CAD build for the part. Positions are in the model's coordinates, mm. A direction names the side the tool comes from. Coordinates: 2 decimals unless noted, no trailing zeros. Order: outer loops, then holes, each group sorted by start corner. A loop starts at its lowest first (then second) coordinate and runs counter-clockwise, first axis right, second up. Notation, with made-up numbers: M 18.5,51.25 L 69.5,51.25 A23 cw 69.5,79.25 Z; hole C 71,-25.5 d9. An arc over 180 degrees is marked long. One line per item, written item: value.
from build123d import *

# Parameters (mm, degrees)
SKETCH1_W                = 66.5
SKETCH1_H                = 180
BOSS_EXTRUDE1_DEPTH      = 180
SKETCH3_W                = 160
SKETCH3_H                = 160
CUT_EXTRUDE1_DEPTH       = 180
SKETCH8_W                = 66.5
SKETCH8_H                = 40
BOSS_EXTRUDE2_DEPTH      = 5
SKETCH10_W               = 66.5
SKETCH10_H               = 40
BOSS_EXTRUDE3_DEPTH      = 5
SKETCH5_R                = 14
CUT_EXTRUDE3_DEPTH       = 10
CUT_EXTRUDE5_DEPTH       = 5
CUT_EXTRUDE6_START       = -5
CUT_EXTRUDE6_DEPTH       = 5
SKETCH12_W               = 66.5
SKETCH12_H               = 40
BOSS_EXTRUDE8_DEPTH      = 5
SKETCH15_R               = 14
CUT_EXTRUDE7_DEPTH       = 200
SKETCH7_R                = 14
CORTE_EXTRUS_O1_DEPTH    = 10
SKETCH13_W               = 66.5
SKETCH13_H               = 40
RESSALTO_EXTRUS_O1_DEPTH = 5


with BuildPart() as part:
    # Sketch1 → Boss-Extrude1 (new body)
    with BuildSketch(Plane.XY):
        with Locations((33.25, 90)):
            Rectangle(SKETCH1_W, SKETCH1_H)
    extrude(amount=BOSS_EXTRUDE1_DEPTH)

    # Sketch3 → Cut-Extrude1 (cut)
    with BuildSketch(Plane.ZY):
        with Locations((90, 90)):
            Rectangle(SKETCH3_W, SKETCH3_H)
    extrude(amount=-CUT_EXTRUDE1_DEPTH, mode=Mode.SUBTRACT)

    # Sketch8 → Boss-Extrude2 (add)
    with BuildSketch(Plane.XY.offset(10)):
        with Locations((33.25, 150)):
            Rectangle(SKETCH8_W, SKETCH8_H)
    extrude(amount=BOSS_EXTRUDE2_DEPTH)

    # Sketch10 → Boss-Extrude3 (add)
    with BuildSketch(Plane(origin=(0, 0, 170), x_dir=(-1, 0, 0), z_dir=(0, 0, -1))):
        with Locations((-33.25, 150)):
            Rectangle(SKETCH10_W, SKETCH10_H)
    extrude(amount=BOSS_EXTRUDE3_DEPTH)

    # Sketch5 → Cut-Extrude3 (cut)
    with BuildSketch(Plane(origin=(0, 180, 0), x_dir=(1, 0, 0), z_dir=(0, 1, 0))):
        with Locations(Location((49.5, -90, 0), (0, 0, 270))):
            Circle(SKETCH5_R)
    extrude(amount=-CUT_EXTRUDE3_DEPTH, mode=Mode.SUBTRACT)

    # Sketch9 → Cut-Extrude5 (cut)
    with BuildSketch(Plane.XY.offset(15)):
        with BuildLine():
            Line((60.5, 164.5), (7.5, 164.5))
            ThreePointArc((7.5, 164.5), (5.378679656, 163.621320344), (4.5, 161.5))
            Line((4.5, 161.5), (4.5, 138.5))
            ThreePointArc((4.5, 138.5), (5.378679656, 136.378679656), (7.5, 135.5))
            Line((7.5, 135.5), (60.5, 135.5))
            ThreePointArc((60.5, 135.5), (62.621320344, 136.378679656), (63.5, 138.5))
            Line((63.5, 138.5), (63.5, 161.5))
            ThreePointArc((63.5, 161.5), (62.621320344, 163.621320344), (60.5, 164.5))
        make_face()
    extrude(amount=-CUT_EXTRUDE5_DEPTH, mode=Mode.SUBTRACT)

    # Sketch11 → Cut-Extrude6 (cut)
    with BuildSketch(Plane(origin=(0, 0, 165), x_dir=(-1, 0, 0), z_dir=(0, 0, -1)).offset(CUT_EXTRUDE6_START)):
        with BuildLine():
            Line((-60.5, 164.5), (-7, 164.5))
            ThreePointArc((-7, 164.5), (-4.878679656, 163.621320344), (-4, 161.5))
            Line((-4, 161.5), (-4, 138.5))
            ThreePointArc((-4, 138.5), (-4.878679656, 136.378679656), (-7, 135.5))
            Line((-7, 135.5), (-60.5, 135.5))
            ThreePointArc((-60.5, 135.5), (-62.621320344, 136.378679656), (-63.5, 138.5))
            Line((-63.5, 138.5), (-63.5, 161.5))
            ThreePointArc((-63.5, 161.5), (-62.621320344, 163.621320344), (-60.5, 164.5))
        make_face()
    extrude(amount=CUT_EXTRUDE6_DEPTH, mode=Mode.SUBTRACT)

    # Sketch12 → Boss-Extrude8 (add)
    with BuildSketch(Plane.XZ.offset(-170)):
        with Locations((33.25, 89.833476808)):
            Rectangle(SKETCH12_W, SKETCH12_H)
        with BuildLine():
            Line((60.5, 75.333476808), (7, 75.333476808))
            ThreePointArc((7, 75.333476808), (4.878679656, 76.212156465), (4, 78.333476808))
            Line((4, 78.333476808), (4, 101.333476808))
            ThreePointArc((4, 101.333476808), (4.878679656, 103.454797152), (7, 104.333476808))
            Line((7, 104.333476808), (60.5, 104.333476808))
            ThreePointArc((60.5, 104.333476808), (62.621320344, 103.454797152), (63.5, 101.333476808))
            Line((63.5, 101.333476808), (63.5, 78.333476808))
            ThreePointArc((63.5, 78.333476808), (62.621320344, 76.212156465), (60.5, 75.333476808))
        make_face(mode=Mode.SUBTRACT)
    extrude(amount=BOSS_EXTRUDE8_DEPTH)

    # Sketch15 → Cut-Extrude7 (cut)
    with BuildSketch(Plane(origin=(0, 0, 0), x_dir=(-1, 0, 0), z_dir=(0, 0, -1))):
        with Locations((-17, 150)):
            Circle(SKETCH15_R)
    extrude(amount=-CUT_EXTRUDE7_DEPTH, mode=Mode.SUBTRACT)

    # Sketch7 → Corte-extrusão1 (cut)
    with BuildSketch(Plane.XZ):
        with Locations(Location((49.5, 43, 0), (0, 0, 270))):
            Circle(SKETCH7_R)
        with Locations(Location((49.5, 137, 0), (0, 0, 270))):
            Circle(SKETCH7_R)
    extrude(amount=-CORTE_EXTRUS_O1_DEPTH, mode=Mode.SUBTRACT)

    # Sketch13 → Ressalto-extrusão1 (add)
    # profile 1 of 2: a face of its own
    with BuildSketch(Plane(origin=(0, 10, 0), x_dir=(1, 0, 0), z_dir=(0, 1, 0))):
        with Locations((33.25, -43)):
            Rectangle(SKETCH13_W, SKETCH13_H)
        with BuildLine():
            Line((7, -57.5), (60.5, -57.5))
            ThreePointArc((60.5, -57.5), (62.621320344, -56.621320344), (63.5, -54.5))
            Line((63.5, -54.5), (63.5, -31.5))
            ThreePointArc((63.5, -31.5), (62.621320344, -29.378679656), (60.5, -28.5))
            Line((60.5, -28.5), (7, -28.5))
            ThreePointArc((7, -28.5), (4.878679656, -29.378679656), (4, -31.5))
            Line((4, -31.5), (4, -54.5))
            ThreePointArc((4, -54.5), (4.878679656, -56.621320344), (7, -57.5))
        make_face(mode=Mode.SUBTRACT)
    # profile 2 of 2: a face of its own
    with BuildSketch(Plane(origin=(0, 10, 0), x_dir=(1, 0, 0), z_dir=(0, 1, 0))):
        with Locations((33.25, -137)):
            Rectangle(SKETCH13_W, SKETCH13_H)
        with BuildLine():
            Line((7, -151.5), (60.5, -151.5))
            ThreePointArc((60.5, -151.5), (62.621320344, -150.621320344), (63.5, -148.5))
            Line((63.5, -148.5), (63.5, -125.5))
            ThreePointArc((63.5, -125.5), (62.621320344, -123.378679656), (60.5, -122.5))
            Line((60.5, -122.5), (7, -122.5))
            ThreePointArc((7, -122.5), (4.878679656, -123.378679656), (4, -125.5))
            Line((4, -125.5), (4, -148.5))
            ThreePointArc((4, -148.5), (4.878679656, -150.621320344), (7, -151.5))
        make_face(mode=Mode.SUBTRACT)
    extrude(amount=RESSALTO_EXTRUS_O1_DEPTH)


solid = part.part
Q1. Mould opens along Z. For faces 1 (the face through (35.83, 4.93, 140.03)), 2 (the face through (33, 180, 89)) say: released by +Z, released by -Z, zero draft, split by the parting line, or undercut.
Recorded:
face 1: undercut
face 2: zero draft
Q2. Slice it at D-D (x = 49.5). Give the number of separate pieces and of enclosed holes in the cut face, plus the area to 4 significant figures.
Recorded:
separate pieces: 3
enclosed holes: 0
area: 6,235 mm^2
Q3. Slice it at B-B (y = 150). List the corners of the cut face in (x, z), plus the area to 3 significant figures.
Recorded:
outline: M 0,0 L 3,0 L 3,15 L 0,15 Z; M 0,165 L 3,165 L 3,180 L 0,180 Z; M 31,0 L 66.5,0 L 66.5,15 L 63.5,15 L 63.5,10 L 31,10 Z; M 31,170 L 63.5,170 L 63.5,165 L 66.5,165 L 66.5,180 L 31,180 Z
area: 830 mm^2
Q4. Slice it at A-A (y = 65.5). List the corners of the cut face in (x, z).
Recorded:
outline: M 0,0 L 66.5,0 L 66.5,10 L 0,10 Z; M 0,170 L 66.5,170 L 66.5,180 L 0,180 Z
Q5. Slice it at C-C (z = 48.5). List the corners of the cut face in (x, y).
Recorded:
outline: M 0,0 L 36.63,0 L 36.63,10 L 4,10 L 4,15 L 0,15 Z; M 0,170 L 66.5,170 L 66.5,180 L 0,180 Z; M 62.37,0 L 66.5,0 L 66.5,15 L 63.5,15 L 63.5,10 L 62.37,10 Z
Q6. Drill centre lines: line 1 along Z through (x, y) = (49.5, 2.5); line 2 along Z through (x, y) = (37, 166); line 3 along Z through (x, y) = (49, 82). Where is each one in solid material? Low to high.
Recorded:
line 1: z = 0 to 29, 57 to 123, 151 to 180
line 2: z = 0 to 15, 69.83 to 75.33, 104.33 to 109.83, 165 to 180
line 3: z = 0 to 10, 170 to 180
Q7. Which spindle directions (+Z, -Z, +X, -X, +Y, -Y) get a long thin tool onto all of the face, cutting with end or side? Do faces 3 (the face through (63.5, 12, 137)), 4 (the face through (34, 130, 168)). Say none if no direction does.
Recorded:
face 3: none
face 4: +X, -X
